Input: part model. Units: mm. Frame: model coordinates. Face numbers are marked on the shaded views. A direction names the side the tool comes from. Round coordinates to 2 decimals unless told otherwise and drop trailing zeros. Loops run counter-clockwise (first coordinate to the right, second up) from the corner with the lowest first, then second, coordinate; pieces in that order, holes last.
1) Draft query along Z for the marked faces 1, 2 and 3. Return one class per face: pulls with the +Z half, pulls with the -Z half, needs draft (parallel to the pull), parting line crosses it, or undercut.
2) Section B-B, the plane x = 100. Return loops of the section in (y, z).
3) Section D-D, the plane y = 29. Return loops of the section in (x, z).
4) Ray query, line 1 along Z through (x, y) = (66, 6); line 2 along Y through (x, z) = (100, 36.25); line 3 along X through (y, z) = (-11.5, 21.5). Return the intervals inside material, ascending.
5) Section C-C, the plane z = 34.5. Return loops of the section in (x, y), and give its area (3 significant figures).
6) Section A-A, the plane y = -8. Return loops of the section in (x, z).
7) Access query for the marked faces 4 and 5. Directions: +Z, -Z, +X, -X, +Y, -Y. A direction counts if a zero-diameter tool reaches every point of the face in a straight line with its end or side. Return the directions, or none.
from build123d import *

# Parameters (mm, degrees)
BOSS_EXTRUDE1_DEPTH      = 40
BOSS_EXTRUDE1_DEPTH_BACK = 40
SKETCH1_W                = 120
SKETCH1_H                = 77
CUT_EXTRUDE1_DEPTH       = 100
CUT_EXTRUDE1_DEPTH_BACK  = 100
SKETCH2_W                = 80
SKETCH2_H                = 61
CUT_EXTRUDE2_DEPTH       = 100
CUT_EXTRUDE2_DEPTH_BACK  = 100
SKETCH3_R                = 10


with BuildPart() as part:
    # Sketch1 → Boss-Extrude1 (new, two sides: drawn at the far end of the back side and taken through both)
    with BuildSketch(Plane(origin=(0, 0, 0), x_dir=(1, 0, 0), z_dir=(0, 1, 0)).offset(-BOSS_EXTRUDE1_DEPTH_BACK)):
        with Locations((60, 0)):
            Rectangle(SKETCH1_W, SKETCH1_H)
    extrude(amount=BOSS_EXTRUDE1_DEPTH + BOSS_EXTRUDE1_DEPTH_BACK)

    # Sketch2 → Cut-Extrude1 (cut, two sides: drawn at the far end of the back side and taken through both)
    with BuildSketch(Plane(origin=(0, 0, 0), x_dir=(1, 0, 0), z_dir=(0, 1, 0)).offset(-CUT_EXTRUDE1_DEPTH_BACK)):
        with Locations((80, 0)):
            Rectangle(SKETCH2_W, SKETCH2_H)
    extrude(amount=CUT_EXTRUDE1_DEPTH + CUT_EXTRUDE1_DEPTH_BACK, mode=Mode.SUBTRACT)

    # Sketch3 → Cut-Extrude2 (cut, two sides: drawn at the far end of the back side and taken through both)
    with BuildSketch(Plane.XY.offset(-CUT_EXTRUDE2_DEPTH_BACK)):
        with Locations(Location((100, 0, 0), (0, 0, 180))):
            Circle(SKETCH3_R)
    extrude(amount=CUT_EXTRUDE2_DEPTH + CUT_EXTRUDE2_DEPTH_BACK, mode=Mode.SUBTRACT)


solid = part.part
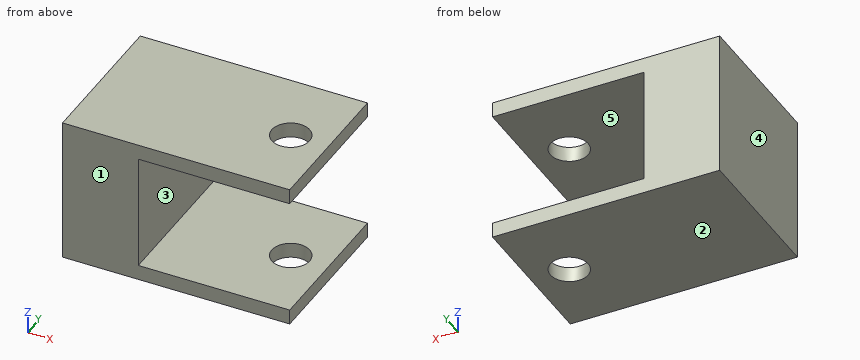
Final values:
1. face 1: needs draft
1. face 2: pulls with the -Z half
1. face 3: undercut
2. outline: (-40, -38.5) - (-10, -38.5) - (-10, -30.5) - (-40, -30.5) - close; (-40, 30.5) - (-10, 30.5) - (-10, 38.5) - (-40, 38.5) - close; (10, -38.5) - (40, -38.5) - (40, -30.5) - (10, -30.5) - close; (10, 30.5) - (40, 30.5) - (40, 38.5) - (10, 38.5) - close
3. outline: (0, -38.5) - (120, -38.5) - (120, -30.5) - (40, -30.5) - (40, 30.5) - (120, 30.5) - (120, 38.5) - (0, 38.5) - close
4. line 1: z = -38.5 to -30.5, 30.5 to 38.5
4. line 2: y = -40 to -10, 10 to 40
4. line 3: x = 0 to 40
5. outline: (0, -40) - (120, -40) - (120, 40) - (0, 40) - close; hole circle Ø20 at (100, 0)
5. area: 9,290 mm2
6. outline: (0, -38.5) - (94, -38.5) - (94, -30.5) - (40, -30.5) - (40, 30.5) - (94, 30.5) - (94, 38.5) - (0, 38.5) - close; (106, -38.5) - (120, -38.5) - (120, -30.5) - (106, -30.5) - close; (106, 30.5) - (120, 30.5) - (120, 38.5) - (106, 38.5) - close
7. face 4: +Z, -Z, -X, +Y, -Y
7. face 5: +X, +Y, -Y
